Here's how the part is built. I have some questions about the finished solid (model axes, mm). A direction names the side the tool comes from. Coordinates: 2 decimals unless noted, no trailing zeros. Write each loop counter-clockwise with the first axis right and the second up, starting at its lowest first coordinate (ties: lowest second). Pieces come first, ordered by that corner, then holes. Notation, with made-up numbers: (89.25, -2.5) - (117.25, -2.5) arc R23 cw to (117.25, 31.5) - close; hole circle Ø9 at (-8.75, -10.5). An arc over 180 degrees is marked (long way). Answer in a Markdown table with one row per item. Add a question column.
Item 1: If I drill on probe 1 along X at (y, z) = (3.8, 0); probe 2 along Z at (x, y) = (116, 3); probe 3 along X at (y, z) = (-4, 0.5), over which ranges is the centre line in solid material (lowest first)? Write a range as from..to.
Item 2: I'm going to push flat-ended pins straight in: pin 1 (3.5 mm diameter, centred on x = 115, y = 0, fed in from +Z); pin 2 (1 mm diameter, centred on x = 53.5, y = 4.5, fed in from +Z); pin 3 (3.5 mm diameter, centred on x = 116, z = 0, fed in from +Y). Where does each tip first touch, or does it pass through?
Item 3: Which directions (+Z, -Z, +X, -X, +Y, -Y) give clear straight access to the entire face, cutting with the end or side of a thin tool? Please do faces 1 (the face through (116, 0, -6)), 2 (the face through (-1, 2.1, 0)), 3 (the face through (116, -6, 0)), 4 (the face through (12.5, 3, 5)).
Item 4: We'd pull the mould along Y, two halves only. Please class faces 5 (the face through (118.018, 2.998, -0.448)), 6 (the face through (6.162, -6.035, 5.985)), 7 (the face through (2.107, 1.035, -1.827)): +Y half, -Y half, draft (parallel to the pull), parting line (faces both ways), or undercut.
Item 5: Imagine slicing it at A-A (x = 8). Please give me the cut outline in (y, z), plus the area to 3 significant figures.
Autodesk Inventor part; units mm, degrees
ref_plane "BODY_N_XY" through (121, 0, 0) normal (0, 0, 1) x (1, 0, 0)
ref_plane "BODY_N_YZ" through (121, 0, 0) normal (1, 0, 0) x (0, 1, 0)
ref_plane "BODY_N_ZX" through (121, 0, 0) normal (0, 1, 0) x (0, 0, 1)
sketch "Sketch_8" plane through (0, 0, 0) normal (0, 0, 1) x (1, 0, 0)
  line L0 (0, 0) -> (-8, 0)
  line L1 (-8, 0) -> (-8, 4.4585)
  line L2 (-8, 4.4585) -> (-7.4585, 5)
  line L3 (-7.4585, 5) -> (0, 5)
  line L4 (0, 5) -> (0, 0)
  line L5 (0, 0) -> (-8, 0)
revolve "Revolution1" add sketch "Sketch_8" angle 360 about axis through (0, 0, 0) along (1, 0, 0)
thread "Thread1"
sketch "Sketch_9" plane through (0, 0, 0) normal (1, 0, 0) x (0, 0, -1)
  line L0 (-7.5, 4) -> (-7.5, -4)
  arc A0 (-7.5, -4) -> (-4, -7.5) centre (0, 0) ccw
  line L1 (-4, -7.5) -> (4, -7.5)
  arc A1 (4, -7.5) -> (7.5, -4) centre (0, 0) ccw
  line L2 (7.5, -4) -> (7.5, 4)
  arc A2 (7.5, 4) -> (4, 7.5) centre (0, 0) ccw
  line L3 (4, 7.5) -> (-4, 7.5)
  arc A3 (-4, 7.5) -> (-7.5, 4) centre (0, 0) ccw
extrude "Extrusion1" add sketch "Sketch_9" along normal blind 12.5
sketch "Sketch_6" plane through (12.5, 0, 0) normal (1, 0, 0) x (0, 0, -1)
  circle A0 centre (0, 0) radius 5.5
extrude "Extrusion2" add sketch "Sketch_6" along normal blind 99
sketch "Sketch_10" plane through (111.5, 0, 0) normal (1, 0, 0) x (0, 0, -1)
  line L0 (-6, 3.6056) -> (-6, -3.6056)
  arc A0 (-6, -3.6056) -> (-3.6056, -6) centre (0, 0) ccw
  line L1 (-3.6056, -6) -> (3.6056, -6)
  arc A1 (3.6056, -6) -> (6, -3.6056) centre (0, 0) ccw
  line L2 (6, -3.6056) -> (6, 3.6056)
  arc A2 (6, 3.6056) -> (3.6056, 6) centre (0, 0) ccw
  line L3 (3.6056, 6) -> (-3.6056, 6)
  arc A3 (-3.6056, 6) -> (-6, 3.6056) centre (0, 0) ccw
extrude "Extrusion3" add sketch "Sketch_10" along normal blind 9.5
sketch "Sketch5" plane through (0, 7.5, 4) normal (0, 1, 0) x (1, 0, 0)
  point P0 (8, 4)
hole "Hole1" at (8, 7.5, 0) direction (0, -1, 0) diameter 4.134 depth 5.5 tip angle 150 countersink diameter 5 countersink angle 90
sketch "Sketch6" plane through (111.5, 6, 3.6056) normal (0, 1, 0) x (1, 0, 0)
  point P0 (4.5, 3.6056)
hole "Hole2" at (116, 6, 0) direction (0, -1, 0) diameter 4.134 depth 5.5 tip angle 150 countersink diameter 5 countersink angle 90
sketch "Sketch_26" plane through (-8, 0, 0) normal (1, 0, 0) x (0, 0, -1)
  line L0 (-2.4249, 0) -> (-1.2124, -2.1)
  line L1 (-1.2124, -2.1) -> (1.2124, -2.1)
  line L2 (1.2124, -2.1) -> (2.4249, 0)
  line L3 (2.4249, 0) -> (1.2124, 2.1)
  line L4 (1.2124, 2.1) -> (-1.2124, 2.1)
  line L5 (-1.2124, 2.1) -> (-2.4249, 0)
extrude "Extrusion4" cut sketch "Sketch_26" along normal blind 20.5
sketch "Sketch_16" plane through (0, 0, 0) normal (0, 0, 1) x (1, 0, 0)
  line L0 (92.5, 0) -> (12.5, 0)
  line L1 (12.5, 0) -> (12.5, 5)
  line L2 (12.5, 5) -> (92.5, 5)
  line L3 (92.5, 5) -> (92.5, 0)
  line L4 (92.5, 0) -> (12.5, 0)
revolve "Revolution2" cut sketch "Sketch_16" angle 360 about axis through (92.5, 0, 0) along (1, 0, 0)
ref_plane "BODY_N_XY" through (121, 0, 0) normal (0, 0, 1) x (1, 0, 0)
ref_plane "BODY_N_YZ" through (121, 0, 0) normal (1, 0, 0) x (0, 1, 0)
ref_plane "BODY_N_ZX" through (121, 0, 0) normal (0, 1, 0) x (0, 0, 1)
ref_plane "BSW1_XY" through (17, 0, 0) normal (1, 0, 0) x (0, 0, -1)
ref_plane "BSW1_YZ" through (17, 0, 0) normal (0, 0, -1) x (0, 1, 0)
ref_plane "BSW1_ZX" through (17, 0, 0) normal (0, 1, 0) x (1, 0, 0)
ref_plane "BSW2_XY" through (107, 0, 0) normal (-1, 0, 0) x (0, 0, -1)
ref_plane "BSW2_YZ" through (107, 0, 0) normal (0, 0, -1) x (0, -1, 0)
ref_plane "BSW2_ZX" through (107, 0, 0) normal (0, -1, 0) x (-1, 0, 0)
ref_plane "RSW1_XY" through (17, -11, 0) normal (1, 0, 0) x (0, 0, -1)
ref_plane "RSW1_YZ" through (17, -11, 0) normal (0, 0, -1) x (0, 1, 0)
ref_plane "RSW1_ZX" through (17, -11, 0) normal (0, 1, 0) x (1, 0, 0)
ref_plane "RSW2_XY" through (107, -11, 0) normal (-1, 0, 0) x (0, 0, -1)
ref_plane "RSW2_YZ" through (107, -11, 0) normal (0, 0, -1) x (0, -1, 0)
ref_plane "RSW2_ZX" through (107, -11, 0) normal (0, -1, 0) x (-1, 0, 0)
ref_plane "body_XY" through (0, 0, 0) normal (1, 0, 0) x (0, 0, -1)
ref_plane "body_YZ" through (0, 0, 0) normal (0, 0, -1) x (0, 1, 0)
ref_plane "body_ZX" through (0, 0, 0) normal (0, 1, 0) x (1, 0, 0)
ref_plane "body2_XY" through (121, 0, 0) normal (-1, 0, 0) x (0, 0, -1)
ref_plane "body2_YZ" through (121, 0, 0) normal (0, 0, -1) x (0, -1, 0)
ref_plane "body2_ZX" through (121, 0, 0) normal (0, -1, 0) x (-1, 0, 0)
ref_plane "rod_XY" through (-28, 0, 0) normal (-1, 0, 0) x (0, 0, -1)
ref_plane "rod_YZ" through (-28, 0, 0) normal (0, 0, -1) x (0, -1, 0)
ref_plane "rod_ZX" through (-28, 0, 0) normal (0, -1, 0) x (-1, 0, 0)
properties part number "CJ2KB10-75Z(0)_BODY" material "ステンレス鋼"
Here are the results:
| question | item | result |
|---|---|---|
| 1 | probe 1 | x = -8..5.93, 10.07..12.5, 92.5..113.93, 118.07..121 |
| 1 | probe 2 | z = -6..-2.07, 2.07..6 |
| 1 | probe 3 | x = -8..12.5, 92.5..121 |
| 2 | pin 1 | stops at z = 6 |
| 2 | pin 2 | stops at z = 3.77 |
| 2 | pin 3 | stops at y = 0.42 |
| 3 | face 1 | -Z, +X, +Y, -Y |
| 3 | face 2 | -X |
| 3 | face 3 | +Z, -Z, +X, -Y |
| 3 | face 4 | none |
| 4 | face 5 | draft |
| 4 | face 6 | -Y half |
| 4 | face 7 | undercut |
| 5 | outline | (-7.5, -4) arc R8.5 ccw to (-4, -7.5) - (4, -7.5) arc R8.5 ccw to (7.5, -4) - (7.5, -2.5) - (7.07, -2.07) - (2, -2.07) - (1.82, -1.38) - (0, -2.42) - (-2.1, -1.21) - (-2.1, 1.21) - (0, 2.42) - (1.82, 1.38) - (2, 2.07) - (7.07, 2.07) - (7.5, 2.5) - (7.5, 4) arc R8.5 ccw to (4, 7.5) - (-4, 7.5) arc R8.5 ccw to (-7.5, 4) - close |
| 5 | area | 167 mm2 |
